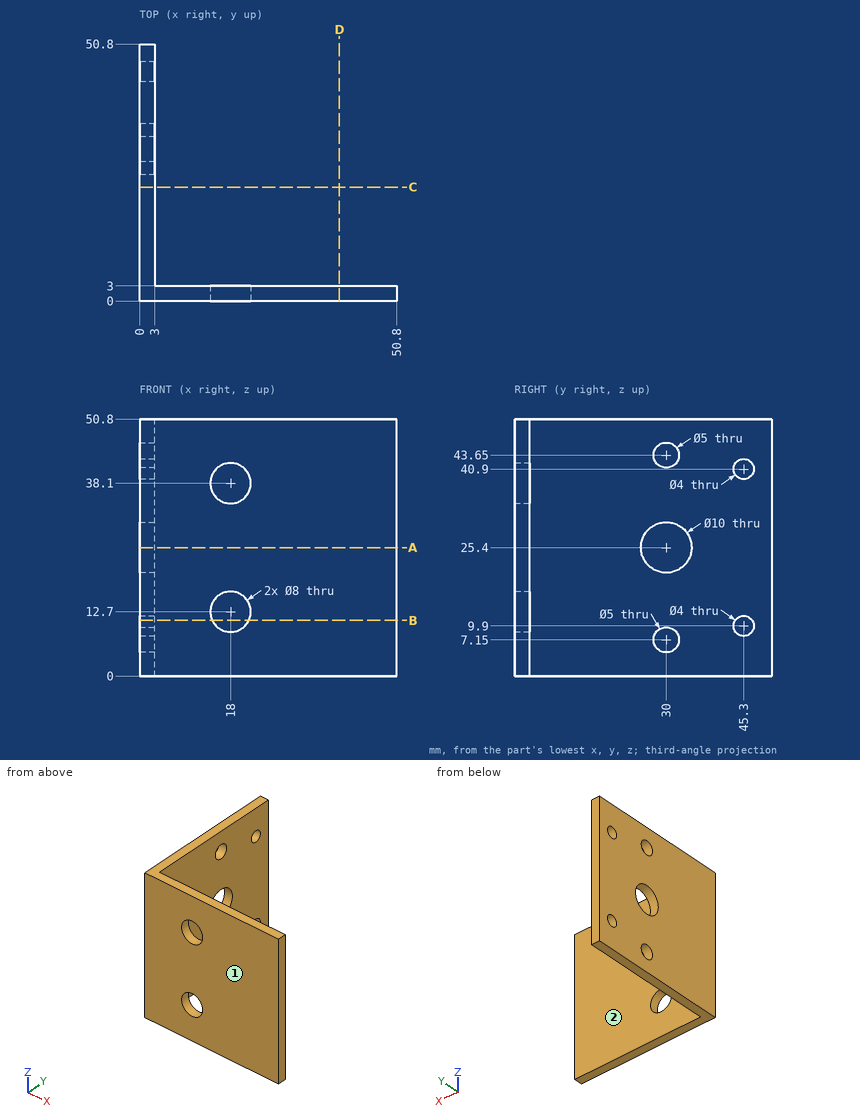
The figure shows three views and two pictorial views of one solid part (mm, origin at its lowest corner). Answer the questions. A direction names the side the tool comes from. Give positions to 0.01 mm unless a question says otherwise; leave off trailing zeros. Loops run counter-clockwise (first coordinate to the right, second up) from the corner with the lowest first, then second, coordinate; pieces in that order, holes last. Notation, with made-up numbers: (89.5, 74) -> (106.5, 74) arc R23 ccw to (106.5, 105) -> close; hole circle Ø4 at (47, 11). An arc over 180 degrees is marked (long way). Use a Markdown table: item, result. Add a question column.
1. Section A-A on z = 25.4 is taken. Determine the outline of the cut face in (x, y), and give its area (3 significant figures).
2. Find the intervals of material crossed by probe 1 along Y at (x, z) = (2.2, 40.9); probe 2 along Y at (x, z) = (2, 7.15); probe 3 along Y at (x, z) = (7.5, 32), in increasing order.
3. Section C-C on y = 22.5 is taken. Determine the outline of the cut face in (x, z).
4. Flat-ended cylindrical pins translate along their axes: pin 1 Ø1 at (x, z) = (45.5, 27.5) entering from +Y; pin 2 Ø6.5 at (y, z) = (30, 7.15) entering from +X. Find the tip coordinate at first contact, or state that the pin passes through.
5. Section B-B on z = 11 is taken. Determine the outline of the cut face in (x, y), and give its area (3 significant figures).
6. For the marked faces 1 and 2, determine the directions among +Z, -Z, +X, -X, +Y, -Y from which every point of the face is accessible in a straight line to the end or side of a thin tool.
Results below:
| question | item | result |
|---|---|---|
| 1 | outline | (0, 0) -> (50.8, 0) -> (50.8, 3) -> (3, 3) -> (3, 25) -> (0, 25) -> close; (0, 35) -> (3, 35) -> (3, 50.8) -> (0, 50.8) -> close |
| 1 | area | 266 mm^2 |
| 2 | probe 1 | y = 0 to 43.3, 47.3 to 50.8 |
| 2 | probe 2 | y = 0 to 27.5, 32.5 to 50.8 |
| 2 | probe 3 | y = 0 to 3 |
| 3 | outline | (0, 0) -> (3, 0) -> (3, 50.8) -> (0, 50.8) -> close |
| 4 | pin 1 | stops at y = 3 |
| 4 | pin 2 | stops at x = 3 |
| 5 | outline | (0, 0) -> (14.38, 0) -> (14.38, 3) -> (3, 3) -> (3, 43.63) -> (0, 43.63) -> close; (0, 46.97) -> (3, 46.97) -> (3, 50.8) -> (0, 50.8) -> close; (21.62, 0) -> (50.8, 0) -> (50.8, 3) -> (21.62, 3) -> close |
| 5 | area | 264 mm^2 |
| 6 | face 1 | +Z, -Z, +X, -X, -Y |
| 6 | face 2 | +Z, -Z, +X, +Y |
